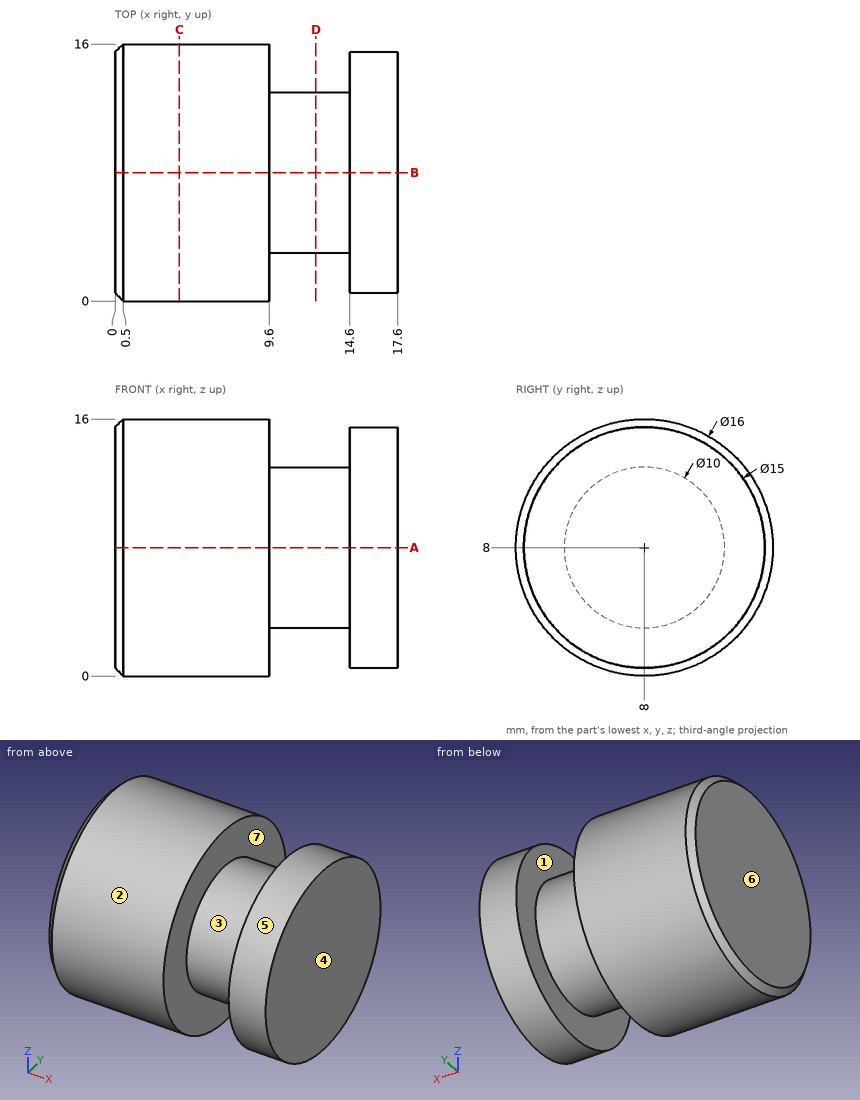
Verification items for this drawing (mm, ordinates from the low corner). A direction names the side the tool comes from. Give positions to 0.01 mm unless a question says otherwise; leave off trailing zeros. Write each loop counter-clockwise with the first axis right and the second up, starting at its lowest first coordinate (ties: lowest second). Pieces come first, ordered by that corner, then holes.
1) Access from +Z, -Z, +X, -X, +Y, -Y to the whole of each face (thin tool, end or side, straight path). Record for the marked faces 5, 6 and 7.
2) Section check D-D, the plane x = 12.5. Record the boundary of the cut face in (y, z).
3) Section check A-A, the plane z = 8. Record the boundary of the cut face in (x, y), and give its area (3 significant figures).
4) Gauge pin test, flat ends, axial feed: pin 1 (1.5 mm diameter, centred on x = 10.5, y = 9, fed in from -Z); pin 2 (4 mm diameter, centred on x = 15.5, y = 3.5, fed in from +Z); pin 3 (1 mm diameter, centred on x = 7, y = 12, fed in from +Z). Record the tip position at first contact, or that the pin passes through.
5) Section check C-C, the plane x = 4. Record the boundary of the cut face in (y, z), and give its area (3 significant figures).
6) Release check for a two-part mould opening along X. For the marked faces 1, 2, 3 and 4 record: pulls with the +X half, pulls with the -X half, needs draft (parallel to the pull), parting line crosses it, or undercut.
7) Material ranges on L1, parallel to X at y = 3.25, z = 10.75; L2, parallel to Y at x = 8.25, z = 15; L3, parallel to Z at x = 14.75, y = 6.5, recorded low to high.
Computed:
1. face 5: +X
1. face 6: +Z, -Z, -X, +Y, -Y
1. face 7: none
2. outline: circle Ø10 at (8, 8)
3. outline: (0, 0.5) - (0.5, 0) - (9.6, 0) - (9.6, 3) - (14.6, 3) - (14.6, 0.5) - (17.6, 0.5) - (17.6, 15.5) - (14.6, 15.5) - (14.6, 13) - (9.6, 13) - (9.6, 16) - (0.5, 16) - (0, 15.5) - close
3. area: 248 mm2
4. pin 1: stops at z = 3.01
4. pin 2: stops at z = 15.07
4. pin 3: stops at z = 15.19
5. outline: circle Ø16 at (8, 8)
5. area: 201 mm2
6. face 1: undercut
6. face 2: needs draft
6. face 3: undercut
6. face 4: pulls with the +X half
7. L1: x = 0 to 9.6, 14.6 to 17.6
7. L2: y = 4.13 to 11.87
7. L3: z = 0.65 to 15.35
